```python
from build123d import *

# Parameters (mm, degrees)
BOSS_EXTRUDE1_DEPTH = 5.08
BOSS_EXTRUDE2_DEPTH = 1.27
SKETCH4_R           = 6.35
BOSS_EXTRUDE3_DEPTH = 9.525
SKETCH5_R           = 4.572
CUT_EXTRUDE1_DEPTH  = 12.7


with BuildPart() as part:
    # Sketch1 → Boss-Extrude1 (new body)
    with BuildSketch(Plane.XY):
        with BuildLine():
            Line((5.715, -8.255), (-5.715, -8.255))
            ThreePointArc((-5.715, -8.255), (-9.307102448, -6.767102448), (-10.795, -3.175))
            Line((-10.795, -3.175), (-10.795, 3.175))
            ThreePointArc((-10.795, 3.175), (-9.307102448, 6.767102448), (-5.715, 8.255))
            Line((-5.715, 8.255), (5.715, 8.255))
            ThreePointArc((5.715, 8.255), (9.307102448, 6.767102448), (10.795, 3.175))
            Line((10.795, 3.175), (10.795, -3.175))
            ThreePointArc((10.795, -3.175), (9.307102448, -6.767102448), (5.715, -8.255))
        make_face()
        with BuildLine():
            Line((3.67, -6), (-3.67, -6))
            ThreePointArc((-3.67, -6), (-7.262102448, -4.512102448), (-8.75, -0.92))
            Line((-8.75, -0.92), (-8.75, 0.92))
            ThreePointArc((-8.75, 0.92), (-7.262102448, 4.512102448), (-3.67, 6))
            Line((-3.67, 6), (3.67, 6))
            ThreePointArc((3.67, 6), (7.262102448, 4.512102448), (8.75, 0.92))
            Line((8.75, 0.92), (8.75, -0.92))
            ThreePointArc((8.75, -0.92), (7.262102448, -4.512102448), (3.67, -6))
        make_face(mode=Mode.SUBTRACT)
    extrude(amount=BOSS_EXTRUDE1_DEPTH)

    # Sketch2 → Boss-Extrude2 (add)
    with BuildSketch(Plane.XY.offset(5.08)):
        with BuildLine():
            Line((5.08, -7.62), (-5.08, -7.62))
            ThreePointArc((-5.08, -7.62), (-8.672102448, -6.132102448), (-10.16, -2.54))
            Line((-10.16, -2.54), (-10.16, 2.54))
            ThreePointArc((-10.16, 2.54), (-8.672102448, 6.132102448), (-5.08, 7.62))
            Line((-5.08, 7.62), (5.08, 7.62))
            ThreePointArc((5.08, 7.62), (8.672102448, 6.132102448), (10.16, 2.54))
            Line((10.16, 2.54), (10.16, -2.54))
            ThreePointArc((10.16, -2.54), (8.672102448, -6.132102448), (5.08, -7.62))
        make_face()
    extrude(amount=BOSS_EXTRUDE2_DEPTH)

    # Sketch4 → Boss-Extrude3 (add)
    with BuildSketch(Plane.XY.offset(6.35)):
        with Locations(Location((0, 0, 0), (0, 0, 180))):
            Circle(SKETCH4_R)
    extrude(amount=BOSS_EXTRUDE3_DEPTH)

    # Sketch5 → Cut-Extrude1 (cut)
    with BuildSketch(Plane.XY.offset(15.875)):
        Circle(SKETCH5_R)
    extrude(amount=-CUT_EXTRUDE1_DEPTH, mode=Mode.SUBTRACT)


solid = part.part
```
Check sheet for the modelled part. Datum: model origin and axes. Units: mm. A direction names the side the tool comes from. Round coordinates to 2 decimals unless told otherwise and drop trailing zeros. Loops run counter-clockwise (first coordinate to the right, second up) from the corner with the lowest first, then second, coordinate; pieces in that order, holes last. Notation, with made-up numbers: (45.5, -0.75) - (94.5, -0.75) arc R28 ccw to (94.5, 32.25) - close; hole circle Ø6 at (79.25, 38). An arc over 180 degrees is marked (long way). Write item = value, one per line. Start each with the question number.
Q1. Thickness scan on L1, parallel to Y at x = 0, z = 11.5; L2, parallel to Z at x = -7.75, y = 1; L3, parallel to Z at x = 4.5, y = 7. Record the ranges inside material, lowest first.
Q2. Section check D-D (x = -8). Record the boundary of the cut face in (y, z).
Q3. Depth check by flat-ended pin: P1, Ø7.5, axis at x = 0, y = 0, coming from the -Z side; P2, Ø4, axis at x = 2.5, z = 7, coming from the +Y side (3 decimals); P3, Ø6, axis at y = 0, z = 11.5, coming from the +X side; P4, Ø6, axis at x = 2.5, y = -2, coming from the -Z side. Enter the tip coordinate at first touch or a pass-through.
Q4. Access from +Z, -Z, +X, -X, +Y, -Y to the whole of each face (thin tool, end or side, straight path). Record for faces 5 (the face through (8.711, -6.092, 5.706)), 6 (the face through (0, 7.62, 6)), 7 (the face through (-7.222, -4.551, 2.504)), 8 (the face through (-7, 0, 6.35)).
Q5. Section check A-A (x = 0). Record the boundary of the cut face in (y, z) (3 decimals), plus the area to 3 significant figures.
Q6. Section check C-C (z = 1.75). Record the boundary of the cut face in (x, y) (3 decimals).
Q7. Section check B-B (y = 0). Record the boundary of the cut face in (x, z) (3 decimals), plus the area to 3 significant figures.
Q8. Release check for a two-part mould opening along Y. For faces 1 (the face through (-9.267, -6.806, 2.504)), 2 (the face through (0, 8, 5.08)), 3 (the face through (9.267, 6.806, 2.504)), 4 (the face through (-8.75, 0, 3)) record: pulls with the +Y half, pulls with the -Y half, needs draft (parallel to the pull), parting line crosses it, or undercut.
Derived:
q1.L1 = -6.35 to -4.57, 4.57 to 6.35
q1.L2 = 5.08 to 6.35
q1.L3 = 0 to 6.35
q2.outline = (-7.71, 0) - (-3.58, 0) - (-3.58, 5.08) - (3.58, 5.08) - (3.58, 0) - (7.71, 0) - (7.71, 5.08) - (6.7, 5.08) - (6.7, 6.35) - (-6.7, 6.35) - (-6.7, 5.08) - (-7.71, 5.08) - close
q3.P1 = through
q3.P2 = 8.255
q3.P3 = 6.35
q3.P4 = 5.08
q4.face_5 = +Z, +X, -Y
q4.face_6 = +Z, +X, -X, +Y
q4.face_7 = -Z
q4.face_8 = +Z
q5.outline = (-8.255, 0) - (-6, 0) - (-6, 5.08) - (-4.572, 5.08) - (-4.572, 15.875) - (-6.35, 15.875) - (-6.35, 6.35) - (-7.62, 6.35) - (-7.62, 5.08) - (-8.255, 5.08) - close; (4.572, 5.08) - (6, 5.08) - (6, 0) - (8.255, 0) - (8.255, 5.08) - (7.62, 5.08) - (7.62, 6.35) - (6.35, 6.35) - (6.35, 15.875) - (4.572, 15.875) - close
q5.area = 64.5 mm^2
q6.outline = (-10.795, -3.175) arc R5.08 ccw to (-5.715, -8.255) - (5.715, -8.255) arc R5.08 ccw to (10.795, -3.175) - (10.795, 3.175) arc R5.08 ccw to (5.715, 8.255) - (-5.715, 8.255) arc R5.08 ccw to (-10.795, 3.175) - close; hole (-8.75, -0.92) arc R5.08 ccw to (-3.67, -6) - (3.67, -6) arc R5.08 ccw to (8.75, -0.92) - (8.75, 0.92) arc R5.08 ccw to (3.67, 6) - (-3.67, 6) arc R5.08 ccw to (-8.75, 0.92) - close
q7.outline = (-10.795, 0) - (-8.75, 0) - (-8.75, 5.08) - (-4.572, 5.08) - (-4.572, 15.875) - (-6.35, 15.875) - (-6.35, 6.35) - (-10.16, 6.35) - (-10.16, 5.08) - (-10.795, 5.08) - close; (4.572, 5.08) - (8.75, 5.08) - (8.75, 0) - (10.795, 0) - (10.795, 5.08) - (10.16, 5.08) - (10.16, 6.35) - (6.35, 6.35) - (6.35, 15.875) - (4.572, 15.875) - close
q7.area = 68.8 mm^2
q8.face_1 = pulls with the -Y half
q8.face_2 = needs draft
q8.face_3 = pulls with the +Y half
q8.face_4 = undercut
